Input: part model. Units: mm. Frame: model coordinates. Face numbers are marked on the shaded views. A direction names the side the tool comes from. Coordinates: 2 decimals unless noted, no trailing zeros. Loops run counter-clockwise (first coordinate to the right, second up) from the corner with the lowest first, then second, coordinate; pieces in that order, holes last. Notation, with made-up numbers: (21, 55.5) - (38, 55.5) arc R19 ccw to (38, 78.5) - close; hole circle Ø3 at (4.5, -12). An arc over 180 degrees is marked (long way). Write item = value, one per line. Start each with the question number.
from build123d import *

# Parameters (mm, degrees)
BASPROSKE_W         = 11
BASPROSKE_H         = 11.25
TOOTHCUT_DEPTH      = 20.342311134
TEETHCUTS_COUNT     = 13
TEETHCUTS_ANGLE     = 332.307692308
BORSKE_R            = 1.5
BORE_DEPTH          = 50.0000508
SKETCH2_R           = 11.5
BOSS_EXTRUDE1_DEPTH = 6
SKETCH4_R           = 3.225
CUT_EXTRUDE1_DEPTH  = 3.8
CUT_EXTRUDE2_START  = -6
SKETCH5_R           = 1.5
CUT_EXTRUDE2_DEPTH  = 6
SKETCH6_R           = 1.725
CUT_EXTRUDE3_DEPTH  = 11.8
CUT_EXTRUDE4_DEPTH  = 6.8
CHAMFER1_SIZE       = 1.5


with BuildPart() as part:
    # BasProSke → Base-Revolve (revolve)
    with BuildSketch(Plane(origin=(0, 0, 0), x_dir=(1, 0, 0), z_dir=(0, 1, 0)), mode=Mode.PRIVATE) as base_revolve_sk:
        with Locations((5.5, 5.625)):
            Rectangle(BASPROSKE_W, BASPROSKE_H)
    revolve(base_revolve_sk.sketch.rotate(Axis((-10, 0, 0), (1, 0, 0)), 180), axis=Axis((-10, 0, 0), (1, 0, 0)))

    # TooCutSke → ToothCut (cut, through all)
    with BuildSketch(Plane(origin=(0, 0, 0), x_dir=(0, 0, -1), z_dir=(1, 0, 0))):
        with BuildLine():
            ThreePointArc((0.95135711, 7.81631599), (0, 7.874), (-0.95135711, 7.81631599))
            ThreePointArc((-0.95135711, 7.81631599), (-1.233506032, 9.58619675), (-2.277442519, 11.043002342))
            ThreePointArc((-2.277442519, 11.043002342), (0, 11.2754), (2.277442519, 11.043002342))
            ThreePointArc((2.277442519, 11.043002342), (1.233506032, 9.58619675), (0.95135711, 7.81631599))
        make_face()
    toothcut = extrude(amount=TOOTHCUT_DEPTH, mode=Mode.SUBTRACT)

    # TeethCuts: ToothCut ×13 about axis
    teethcuts_axis = Axis((-10, 0, 0), (1, 0, 0))
    for i in range(1, TEETHCUTS_COUNT):
        add(toothcut.rotate(teethcuts_axis, i * TEETHCUTS_ANGLE / (TEETHCUTS_COUNT - 1)), mode=Mode.SUBTRACT)

    # BorSke → Bore (cut, symmetric)
    with BuildSketch(Plane(origin=(0, 0, 0), x_dir=(0, 0, -1), z_dir=(1, 0, 0))):
        with Locations(Location((0, 0, 0), (0, 0, 180))):
            Circle(BORSKE_R)
    extrude(amount=BORE_DEPTH, both=True, mode=Mode.SUBTRACT)

    # Sketch2 → Boss-Extrude1 (add)
    with BuildSketch(Plane.ZY):
        Circle(SKETCH2_R)
    extrude(amount=BOSS_EXTRUDE1_DEPTH)

    # Sketch4 → Cut-Extrude1 (cut)
    with BuildSketch(Plane.ZY.offset(6)):
        Circle(SKETCH4_R)
    extrude(amount=-CUT_EXTRUDE1_DEPTH, mode=Mode.SUBTRACT)

    # Sketch5 → Cut-Extrude2 (cut)
    with BuildSketch(Plane.ZY.offset(6).offset(CUT_EXTRUDE2_START)):
        Circle(SKETCH5_R)
    extrude(amount=CUT_EXTRUDE2_DEPTH, mode=Mode.SUBTRACT)

    # Sketch6 → Cut-Extrude3 (cut)
    with BuildSketch(Plane(origin=(0, 0, 0), x_dir=(1, 0, 0), z_dir=(0, 1, 0))):
        with Locations(Location((-2.5, 0, 0), (0, 0, 270))):
            Circle(SKETCH6_R)
    extrude(amount=-CUT_EXTRUDE3_DEPTH, mode=Mode.SUBTRACT)

    # Sketch7 → Cut-Extrude4 (cut)
    with BuildSketch(Plane.ZY.offset(6)):
        Polygon((-2.85, -1.370675016), (-2.85, -5.825), (2.85, -5.825), (2.85, -1.370675016), (1.698712748, -1.370675016), (1.698712748, 0), (-1.698712748, 0), (-1.698712748, -1.370675016), align=None)
    extrude(amount=-CUT_EXTRUDE4_DEPTH, mode=Mode.SUBTRACT)

    # Chamfer1
    chamfer1_edges = [part.edges().sort_by_distance(p)[0] for p in [
        (11, -6.390728401, 9.258568491),
        (11, 10.923095446, -2.692301223),
        (11, -9.961380289, 5.228135685),
        (11, -11.25, 0),
        (11, -9.961380289, -5.228135685),
        (11, -6.390728401, -9.258568491),
        (11, -1.356037653, -11.167974834),
        (11, 3.989304979, -10.51893273),
        (11, 8.420745917, -7.460129905),
        (11, 10.923095446, 2.692301223),
        (11, 8.420745917, 7.460129905),
        (11, 3.989304979, 10.51893273),
        (11, -1.356037653, 11.167974834),
    ]]
    chamfer(chamfer1_edges, length=CHAMFER1_SIZE)


solid = part.part
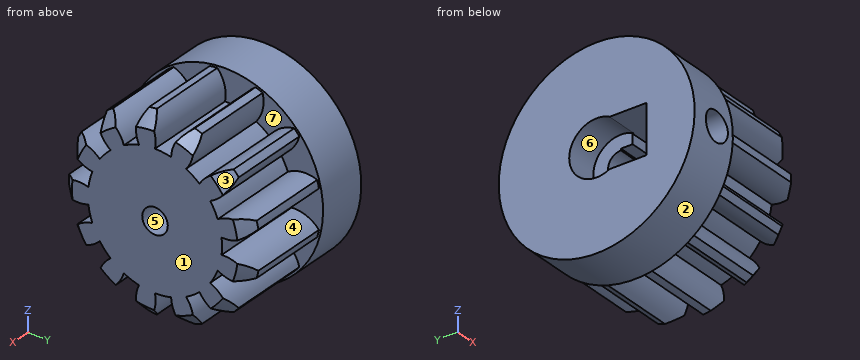
Item 1: Cut plane A-A on z = 0. Return loops of the section in (x, y) (3 decimals).
Item 2: Ray query, line 1 (Z direction, x = -2.5, y = -9.5) (3 decimals); line 2 (Y direction, x = 1, z = 0); line 3 (Z direction, x = 1.5, y = -8.5). Return the intervals inside material, ascending.
Item 3: Cut plane C-C on x = -2.5. Return loops of the section in (y, z) (3 decimals), plus the area to 3 significant figures.
Item 4: Cut plane B-B on y = 0.5. Return loops of the section in (x, z), plus the area to 3 significant figures.
Item 5: Pull-direction query (Z, two-part tool) for the marked faces 1, 2, 3 and 4; classes: pulls with the +Z half, pulls with the -Z half, needs draft (parallel to the pull), parting line crosses it, or undercut.
Item 6: Access query for the marked faces 5, 6 and 7. Directions: +Z, -Z, +X, -X, +Y, -Y. A direction counts if a zero-diameter tool reaches every point of the face in a straight line with its end or side. Return the directions, or none.
Item 7: Cut plane D-D on y = -2.75. Return loops of the section in (x, z).
Item 8: Pin query (flat end, axial travel): pin 1 (3.5 mm diameter, centred on x = -3.5, y = -3.5, fed in from -Z); pin 2 (1.3 mm diameter, centred on x = -0.5, z = 2, fed in from -Y); pin 3 (4 mm diameter, centred on x = 9, z = -4, fed in from -Y); pin 4 (1.8 mm diameter, centred on y = 0, z = 0, fed in from -X) (1 decimal). Return the tip coordinate at first contact, or that it passes through.
Recorded:
q1.outline = (-6, -11.5) - (-4.225, -11.5) - (-4.225, -5.825) - (-6, -5.825) - close; (-6, 3.225) - (-2.2, 3.225) - (-2.2, 1.5) - (11, 1.5) - (11, 7.874) - (0, 7.874) - (0, 11.5) - (-6, 11.5) - close; (-0.775, -11.5) - (0, -11.5) - (0, -11.25) - (9.5, -11.25) - (11, -9.75) - (11, -1.5) - (0.8, -1.5) - (0.8, -5.825) - (-0.775, -5.825) - close
q2.line_1 = -6.481 to -1.725, 1.725 to 6.481
q2.line_2 = -11.25 to -1.5, 1.5 to 7.87
q2.line_3 = -5.57 to -3.17, -1.1 to 1.1, 3.17 to 5.57
q3.outline = (-11.37, -1.725) arc R11.5 ccw (long way) to (-11.37, 1.725) - (-5.825, 1.725) - (-5.825, 2.85) - (-1.509, 2.85) arc R3.225 cw (long way) to (-1.509, -2.85) - (-5.825, -2.85) - (-5.825, -1.725) - close
q3.area = 346 mm²
q4.outline = (-6, -11.49) - (0, -11.49) - (0, -7.86) - (11, -7.86) - (11, -1.41) - (-2.2, -1.41) - (-2.2, -3.19) - (-6, -3.19) - close; (-6, 3.19) - (-2.2, 3.19) - (-2.2, 1.41) - (11, 1.41) - (11, 7.86) - (0, 7.86) - (0, 11.49) - (-6, 11.49) - close
q4.area = 249 mm²
q5.face_1 = needs draft
q5.face_2 = parting line crosses it
q5.face_3 = pulls with the +Z half
q5.face_4 = undercut
q6.face_5 = +X, -X
q6.face_6 = -X
q6.face_7 = +X
q7.outline = (-6, -11.17) - (0, -11.17) - (0, -7.38) - (11, -7.38) - (11, 7.38) - (0, 7.38) - (0, 11.17) - (-6, 11.17) - (-6, 2.85) - (0.8, 2.85) - (0.8, -2.85) - (-6, -2.85) - close
q8.pin_1 = -11.37
q8.pin_2 = -11.42
q8.pin_3 = -10.16
q8.pin_4 = through
